CAD build for the part. Positions are in the model's coordinates, mm. Face numbers are marked on the shaded views. A direction names the side the tool comes from. Give positions to 0.01 mm unless a question says otherwise; leave off trailing zeros. Loops run counter-clockwise (first coordinate to the right, second up) from the corner with the lowest first, then second, coordinate; pieces in that order, holes last. Notation, with made-up numbers: (39, 33.25) -> (50, 33.25) arc R23 ccw to (50, 44.25) -> close; hole circle Ø10 at (17.5, 89). An arc over 180 degrees is marked (long way). Use one line per item in the form item = value.
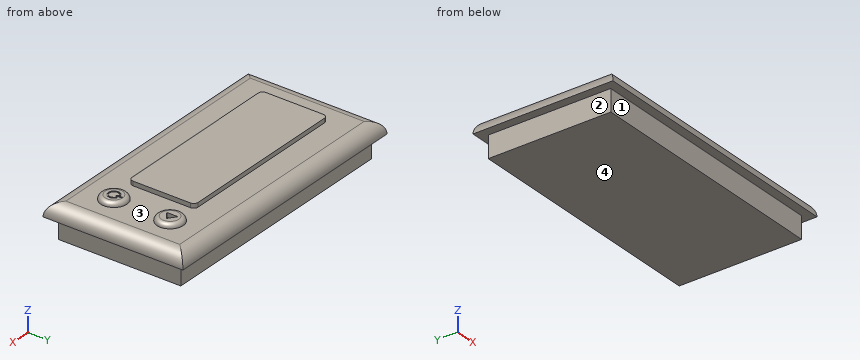
```python
from build123d import *

# Parameters (mm, degrees)
SKETCH1_W           = 58
SKETCH1_H           = 28.1
BOSS_EXTRUDE1_DEPTH = 5
SKETCH2_W           = 62
SKETCH2_H           = 32.1
BOSS_EXTRUDE2_DEPTH = 3
FILLET1_R           = 3
SKETCH3_W           = 40.354739258
SKETCH3_H           = 15.166433462
BOSS_EXTRUDE3_DEPTH = 1
SKETCH3_6_R         = 3.000616935
BOSS_EXTRUDE4_DEPTH = 1
FILLET2_R           = 1
CUT_EXTRUDE2_DEPTH  = 1
CUT_EXTRUDE3_DEPTH  = 0.2
FILLET3_R           = 1


with BuildPart() as part:
    # Sketch1 → Boss-Extrude1 (new body)
    with BuildSketch(Plane.XY):
        Rectangle(SKETCH1_W, SKETCH1_H)
    extrude(amount=BOSS_EXTRUDE1_DEPTH)

    # Sketch2 → Boss-Extrude2 (add)
    with BuildSketch(Plane.XY.offset(5)):
        Rectangle(SKETCH2_W, SKETCH2_H)
    extrude(amount=BOSS_EXTRUDE2_DEPTH)

    # Fillet1
    fillet1_edges = [part.edges().sort_by_distance(p)[0] for p in [
        (0, -16.05, 8),
        (-31, 0, 8),
        (0, 16.05, 8),
        (31, 0, 8),
    ]]
    fillet(fillet1_edges, radius=FILLET1_R - 0.0001)  # a hair under: the kernel refuses the full size

    # Sketch3 → Boss-Extrude3 (add)
    with BuildSketch(Plane.XY.offset(8)):
        with Locations((-4.008748933, 0)):
            Rectangle(SKETCH3_W, SKETCH3_H)
    extrude(amount=BOSS_EXTRUDE3_DEPTH)

    # Sketch3<6> → Boss-Extrude4 (add)
    with BuildSketch(Plane.XY.offset(8)):
        with Locations((22.181744095, 6.447404534)):
            Circle(SKETCH3_6_R)
        with Locations(Location((22.181744095, -6.447404534, 0), (0, 0, 180))):
            Circle(SKETCH3_6_R)
    extrude(amount=BOSS_EXTRUDE4_DEPTH)

    # Fillet2
    fillet2_edges = [part.edges().sort_by_distance(p)[0] for p in [
        (19.18112716, 6.447404534, 9),
        (25.182361031, -6.447404534, 9),
    ]]
    fillet(fillet2_edges, radius=FILLET2_R - 0.0001)  # a hair under: the kernel refuses the full size

    # Sketch4 → Cut-Extrude2 (cut)
    with BuildSketch(Plane.XY.offset(9)):
        Polygon((21.526754794, 7.76375697), (21.526754794, 5.190828819), (23.312816568, 6.477292894), align=None)
    extrude(amount=-CUT_EXTRUDE2_DEPTH, mode=Mode.SUBTRACT)

    # Sketch5 → Cut-Extrude3 (cut)
    with BuildSketch(Plane.XY.offset(9)):
        with BuildLine():
            Line((22.662681188, -5.238974178), (22.559669099, -5.520902001))
            ThreePointArc((22.559669099, -5.520902001), (22.181744095, -7.448021469), (21.803819092, -5.520902001))
            Line((21.803819092, -5.520902001), (21.700807003, -5.238974178))
            ThreePointArc((21.700807003, -5.238974178), (22.181744095, -7.748021469), (22.662681188, -5.238974178))
        make_face()
        with BuildLine():
            Line((22.331744095, -5.86984139), (22.331744095, -4.631238623))
            ThreePointArc((22.331744095, -4.631238623), (22.181744095, -4.625054783), (22.031744095, -4.631238623))
            Line((22.031744095, -4.631238623), (22.031744095, -5.86984139))
            Line((22.031744095, -5.86984139), (22.331744095, -5.86984139))
        make_face()
    extrude(amount=-CUT_EXTRUDE3_DEPTH, mode=Mode.SUBTRACT)

    # Fillet3
    fillet3_edges = [part.edges().sort_by_distance(p)[0] for p in [
        (-24.186118562, 7.583216731, 8.5),
        (-24.186118562, -7.583216731, 8.5),
        (16.168620696, -7.583216731, 8.5),
        (16.168620696, 7.583216731, 8.5),
    ]]
    fillet(fillet3_edges, radius=FILLET3_R)


solid = part.part
```
1. Tool access for the marked faces 1, 2, 3 and 4: list every direction of +Z, -Z, +X, -X, +Y, -Y with a clear straight run to the whole face (end or side of a thin tool).
Result sheet:
face_1 = -Z, +X, -X, -Y
face_2 = -Z, -X, +Y, -Y
face_3 = +Z
face_4 = -Z, +X, -X, +Y, -Y
2. Drop flat-ended pins along their axis: P1, Ø6, axis at x = 7.5, y = -12.5, coming from the +Z side; P2, Ø4, axis at x = 2, z = 1.5, coming from the +Y side; P3, Ø2.5, axis at x = 0.5, z = 2.5, coming from the -Y side. Give the stop position or say it passes through.
Result sheet:
P1 = 8
P2 = 14.05
P3 = -14.05
3. Cut at C-C, the plane z = 3.5. Write the cut outline in (x, y).
Result sheet:
outline = (-29, -14.05) -> (29, -14.05) -> (29, 14.05) -> (-29, 14.05) -> close
4. Drill centre lines: line 1 (X direction, y = 1, z = 5.25); line 2 (X direction, y = -1.5, z = 0.5); line 3 (Y direction, x = 3, z = 2.75). Where is each one in solid material? Low to high.
Result sheet:
line_1 = -30.99 to 30.99
line_2 = -29 to 29
line_3 = -14.05 to 14.05
